Could you check a few things on this drawing? It's one solid part, dimensions in mm from its lowest x, y, z. Give positions to 0.01 mm unless a question says otherwise; leave off trailing zeros. Loops run counter-clockwise (first coordinate to the right, second up) from the corner with the lowest first, then second, coordinate; pieces in that order, holes last. Notation, with made-up numbers: M 53.5,-7.5 L 74.5,-7.5 A19 cw 74.5,12.5 Z; hole C 40,11.25 d3. An arc over 180 degrees is marked long. Answer as CSV lines item,"result". Start each with the question number.
Item 1: I want a section at A-A on y = 8. List the corners of the cut face in (x, z) for me (1 decimal).
Item 2: If we mould it in two halves opening along X, with no side actions, what happens to the marked faces 1, 2 and 3? For each: released by +X, released by -X, zero draft, split by the parting line, or undercut.
Item 3: Will these pins go through, and if not, where does the flat tip stop? P1, Ø1.5, axis at y = 10.5, z = 3, coming from the +X side; P2, Ø1.2, axis at x = 4, z = 3, coming from the +Y side; P3, Ø2, axis at x = 1.5, y = 8.5, coming from the -Z side.
Item 4: If I drill on line 1 along Y through (x, z) = (4, 5.5); line 2 along X through (y, z) = (8.5, 3.25) (1 decimal); line 3 along X through (y, z) = (7.5, 1) (1 decimal), over which ranges is the centre line in solid material (lowest first)? Write a range as from..to.
Item 5: I want a section at B-B on y = 9.75. List the corners of the cut face in (x, z) for me (1 decimal).
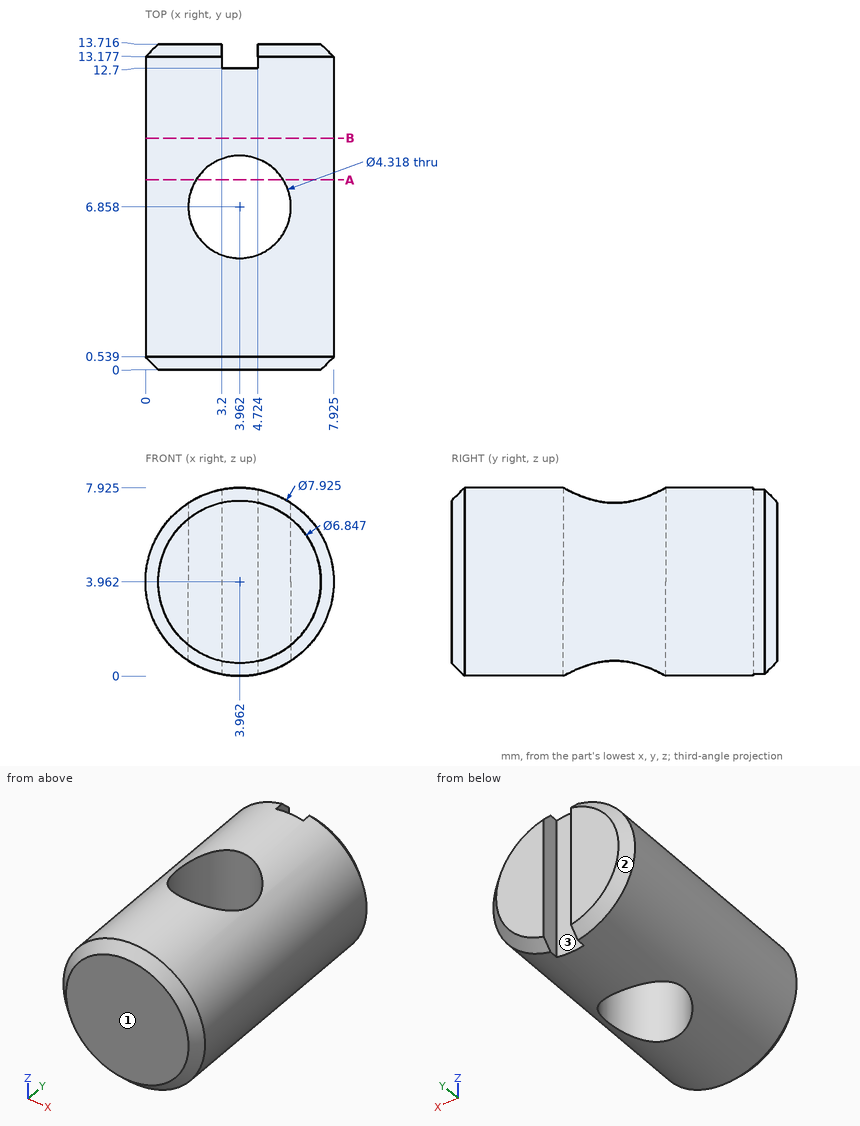
Result:
1,outline,"M 2.1,0.4 L 2.1,7.5 A4 ccw Z; M 5.8,0.4 A4 ccw 5.8,7.5 Z"
2,face 1,"zero draft"
2,face 2,"released by -X"
2,face 3,"undercut"
3,P1,"x = 7.92"
3,P2,"y = 12.7"
3,P3,"z = 0.28"
4,line 1,"0..4.7, 9.02..12.7"
4,line 2,"0.1..2.6, 5.4..7.9"
4,line 3,"1.3..1.9, 6..6.6"
5,outline,"C 4,4 d7.9"
